from build123d import *

# Parameters (mm, degrees)
F1_DEPTH    = 30
F2_T        = -2.5
F3_R        = 5
F4_DEPTH    = 12.6
F5_T1_DEPTH = 70


# Not quite as in the source:
# - a fillet or chamfer that OpenCascade refuses, or shapes differently, is made with other operations: its cross-section is extruded or revolved along the edge and cut away or added


with BuildPart() as f1:
    # F0 (on Top) → F1 (new body)
    with BuildSketch(Plane.XY):
        Polygon((16.1803398875, 5.2573111212), (0, 17.013016167), (-16.1803398875, 5.2573111212), (-10, -13.7638192047), (10, -13.7638192047), align=None)
    extrude(amount=F1_DEPTH)

    # F2
    f2_openings = [f1.faces().sort_by_distance(p)[0] for p in [
        (0, 0, 30),
    ]]
    offset(amount=F2_T, openings=f2_openings)

    # F3 (on face) → F4 (cut)
    with BuildSketch(Plane(origin=(13.0901699437, -4.2532540418, 0), x_dir=(0.3090169944, 0.9510565163, 0), z_dir=(0.9510565163, -0.3090169944, 0))):
        with Locations((0, 18)):
            Circle(F3_R)
    extrude(amount=-F4_DEPTH, mode=Mode.SUBTRACT)

    # F5: fillet of radius 10 on 1 edges, made by hand

    # F5_s2 → F5_t1 (cut)
    with BuildSketch(Plane.YZ.offset(-35)):
        with BuildLine():
            ThreePointArc((-3.7638192047, 30), (-10.8348870166, 27.0710678119), (-13.7638192047, 20))
            Line((-13.7638192047, 20), (-13.7638192047, 30))
            Line((-13.7638192047, 30), (-3.7638192047, 30))
        make_face()
    extrude(amount=F5_T1_DEPTH, mode=Mode.SUBTRACT)


solid = f1.part
Could you check a few things on this model? Use its own coordinates, in mm. A direction names the side the tool comes from. Coordinates: 2 decimals unless noted, no trailing zeros. Loops run counter-clockwise (first coordinate to the right, second up) from the corner with the lowest first, then second, coordinate; pieces in that order, holes last.
1. Imagine slicing it at A-A (z = 4). Please give me the cut outline in (x, y), and give its area (3 significant figures).
2. Imagine slicing it at C-C (z = 17.5). Please give me the cut outline in (x, y), and give its area (3 significant figures).
3. Imagine slicing it at D-D (y = 9). Please give me the cut outline in (x, z), and give its area (3 significant figures).
4. Imagine slicing it at B-B (x = -5). Please give me the cut outline in (y, z).
5. For faces 1 (the face through (0, -13.764, 10)), 2 (the face through (0, -11.264, 14)), which set-ups out of +Z, -Z, +X, -X, +Y, -Y let a thin tool reach every point of the face, with its end or its side?
6. For P1, Ø1.5, axis at x = 10, y = 12, coming from the -Z side; P2, Ø8, axis at y = 10, z = 7, coming from the -X side; P3, Ø1, axis at y = 6, z = 6, coming from the -X side; P4, Ø1.5, axis at y = -2.5, z = 14.5, coming from the +X side, each with a flat end and sliding along its axis, tell me the tip position at first contact or that it passes through.
7. We'd pull the mould along X, two halves only. Please class faces 3 (the face through (13.047, -4.386, 11.457)), 4 (the face through (-13.133, -4.12, 14.79)), 5 (the face through (11.24, -1.86, 13)): released by +X, released by -X, zero draft, split by the parting line, or undercut.
8. I need wall thicknesses on L1, parallel to X at y = 1.5, z = 24; L2, parallel to X at y = -1, z = 9; L3, parallel to Z at x = 12, y = -0.5. Which ranges of each line are inside material? Lowest first, please.
Computed values:
1. outline: (-16.18, 5.26) - (-10, -13.76) - (10, -13.76) - (16.18, 5.26) - (0, 17.01) - close; hole (-13.24, 4.3) - (-8.18, -11.26) - (8.18, -11.26) - (13.24, 4.3) - (0, 13.92) - close
1. area: 227 mm2
2. outline: (-16.18, 5.26) - (-10, -13.76) - (10, -13.76) - (11.55, -8.98) - (9.18, -8.21) - (8.18, -11.26) - (-8.18, -11.26) - (-13.24, 4.3) - (0, 13.92) - (13.24, 4.3) - (12.25, 1.25) - (14.63, 0.48) - (16.18, 5.26) - (0, 17.01) - close
2. area: 202 mm2
3. outline: (-11.03, 0) - (11.03, 0) - (11.03, 30) - (6.78, 30) - (6.78, 2.5) - (-6.78, 2.5) - (-6.78, 30) - (-11.03, 30) - close
3. area: 289 mm2
4. outline: (-13.76, 0) - (13.38, 0) - (13.38, 30) - (10.29, 30) - (10.29, 2.5) - (-11.26, 2.5) - (-11.26, 26.61) arc R10 ccw to (-13.76, 20) - close
5. face 1: +Z, -Z, +X, -X, -Y
5. face 2: +Z
6. P1: passes through
6. P2: stops at x = -15.16
6. P3: stops at x = -15.85
6. P4: stops at x = -10.79
7. face 3: released by +X
7. face 4: released by -X
7. face 5: undercut
8. L1: x = -14.96 to -12.33, 12.33 to 14.96
8. L2: x = -14.15 to -11.52, 11.52 to 14.15
8. L3: z = 0 to 14.19, 21.81 to 30
